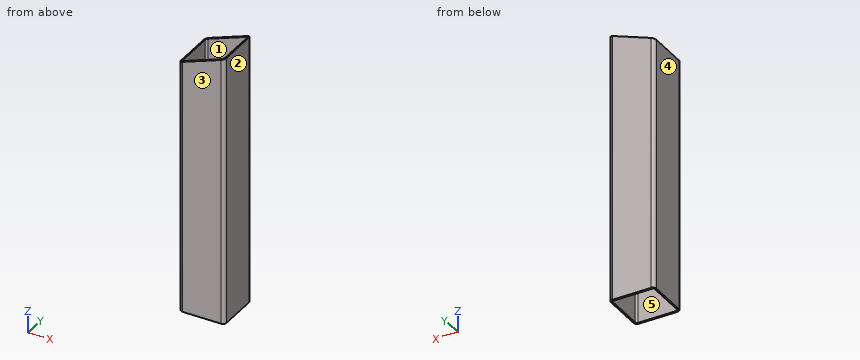
Autodesk Inventor part; units mm, degrees
ref_plane "Start plane" through (0, 0, 0) normal (0, 0, 1) x (1, 0, 0)
ref_plane "End plane" through (0, 0, 1000) normal (0, 0, 1) x (1, 0, 0)
ref_plane "YZ Plane" through (0, 0, 0) normal (1, 0, 0) x (0, 1, 0)
ref_plane "Start plane" through (0, 0, 0) normal (0, 0, 1) x (1, 0, 0)
ref_plane "End plane" through (0, 0, 1000) normal (0, 0, 1) x (1, 0, 0)
sketch "Sketch" plane through (0, 0, 0) normal (0, 0, 1) x (1, 0, 0)
  line L0 (-40, -34) -> (-40, 34)
  line L1 (-34, 40) -> (34, 40)
  line L2 (40, 34) -> (40, -34)
  line L3 (34, -40) -> (-34, -40)
  arc A0 (-40, -34) -> (-34, -40) centre (-34, -34) ccw
  arc A1 (40, 34) -> (34, 40) centre (34, 34) ccw
  arc A2 (-34, 40) -> (-40, 34) centre (-34, 34) ccw
  arc A3 (34, -40) -> (40, -34) centre (34, -34) ccw
  arc A4 (-34, 37) -> (-37, 34) centre (-34, 34) ccw
  line L4 (-34, 37) -> (34, 37)
  arc A5 (37, 34) -> (34, 37) centre (34, 34) ccw
  line L5 (37, 34) -> (37, -34)
  arc A6 (34, -37) -> (37, -34) centre (34, -34) ccw
  line L6 (34, -37) -> (-34, -37)
  arc A7 (-37, -34) -> (-34, -37) centre (-34, -34) ccw
  line L7 (-37, -34) -> (-37, 34)
  line L8 (0, 57.7397) -> (0, -57.7397) construction
  line L9 (-1453.6197, 0) -> (290.3864, 0) construction
  dimension "d7" = 6
  dimension "d9" = 80
  dimension "d11" = 80
  dimension "d12" = 3
  dimension "d15" = 40
  dimension "d16" = 40
extrude "Body" add sketch "Sketch" along normal up to surface (1000 mm away) from surface at 0
sketch "Sketch3" plane through (0, 0, 0) normal (0, 0, 1) x (1, 0, 0)
  line L0 (0, 0) -> (10, 0)
ref_plane "Work Plane3" through (0, 0, 0) normal (0, -1, 0) x (1, 0, 0)
sketch "Sketch5" plane through (0, 0, 0) normal (0, 1, 0) x (-1, 0, 0)
  line L0 (-40, 0) -> (-40, 1000)
  line L1 (40, 0) -> (40, 1000)
  line L2 (40, 0) -> (40, 1000)
  line L3 (40, 458.04) -> (415, 458.04) construction
  line L4 (-5.663, 479.3796) -> (835.663, 479.3796) construction
  arc A0 (-5.663, 479.3796) -> (415, 380) centre (415, 1320) ccw construction
  line L5 (-55, 559.2385) -> (885, 559.2385) construction
  arc A1 (-55, 559.2385) -> (-5.663, 479.3796) centre (34.3, 559.2385) ccw construction
  arc A2 (835.663, 479.3796) -> (885, 559.2385) centre (795.7, 559.2385) ccw
  line L6 (-55, 559.2385) -> (-55, 599.2385)
  line L7 (885, 559.2385) -> (885, 599.2385)
  line L8 (-55, 599.2385) -> (415, 599.2385) construction
  line L9 (415, 599.2385) -> (415, 0)
  arc A3 (415, 380) -> (835.663, 479.3796) centre (415, 1320) ccw
  line L10 (415, 599.2385) -> (885, 599.2385)
  point P0 (0, 0)
  dimension "d22" = 375
  dimension "d24" = 940
  dimension "d25" = 89.3
  dimension "d26" = 40
  dimension "d27" = 940
  dimension "d28" = 380
  dimension "d30" = 458.04
sketch "Sketch6" plane through (0, 0, 0) normal (0, 1, 0) x (-1, 0, 0)
  line L0 (40, 0) -> (40, 1000)
  line L1 (40, 0) -> (40, 1000)
  line L2 (-40, 0) -> (-40, 1000)
  line L3 (-40, 0) -> (-40, 1000)
  line L4 (34, 1000) -> (40, 1000)
  line L5 (40, 1000) -> (-40, 1000)
  arc A0 (-5.663, 479.3796) -> (415, 380) centre (415, 1320) ccw construction
  line L6 (40, 447.8824) -> (-40, 477)
  point P0 (0, 0)
  dimension "d34" = 110
  dimension "d36" = 477
extrude "Extrusion2" cut sketch "Sketch6" along normal through all both and the other way through all
sketch "Sketch4" plane through (0, 0, 0) normal (0, -1, 0) x (1, 0, 0)
  line L0 (-1453.3712, 0) -> (288.8952, 0)
  line L1 (-1453.3712, 1000) -> (288.8952, 1000)
  dimension "d18" = 1000
equation "\"d7\" = G_IR"
equation "\"d9\" = G_W"
equation "\"d11\" = G_H"
equation "\"d12\" = G_T"
equation "\"d15\" = 0.5 * d9"
equation "\"d16\" = 0.5 * d11"
equation "\"d3\" = G_L"
equation "\"d22\" = 0.5 * Diam_of_legs_center"
equation "\"d24\" = d27"
equation "\"d25\" = 0.095 * d27"
equation "\"d27\" = MAIN_filter_diam"
equation "\"G_W\" = 80"
equation "\"G_H\" = 80"
equation "\"G_T\" = 3"
equation "\"G_IR\" = 6"
equation "\"G_L\" = d18"
equation "\"G_OFFSET_START\" = 0"
equation "\"G_OFFSET_END\" = 0"
equation "\"MAIN_filter_diam\" = 940"
properties part number "SLM 1692 Leg tube" material "Steel, Mild"
Could you check a few things on this model? Use its own coordinates, in mm. Face numbers are marked on the shaded views. A direction names the side the tool comes from. Coordinates: 2 decimals unless noted, no trailing zeros. Order: outer loops, then holes, each group sorted by start corner. A loop starts at its lowest first (then second) coordinate and runs counter-clockwise, first axis right, second up. Notation, with made-up numbers: M -35,85 L 6,85 A9 ccw 6,102 Z; hole C -24,13 d6. An arc over 180 degrees is marked long. Use a Markdown table: item, result. Add a question column.
Q1. I want a section at B-B on z = 266.5. List the corners of the cut face in (x, y) for me.
Q2. Which directions (+Z, -Z, +X, -X, +Y, -Y) give clear straight access to the entire face, cutting with the end or side of a thin tool? Please do the marked faces 1 and 2.
Q3. We'd pull the mould along X, two halves only. Please class the marked faces 3, 4 and 5: pulls with the +X half, pulls with the -X half, needs draft (parallel to the pull), parting line crosses it, or undercut.
Q4. I want a section at C-C on x = 20.5. List the corners of the cut face in (y, z) for me, then the cut area to 3 significant figures.
Q5. I want a section at A-A on y = 5.5. List the corners of the cut face in (x, z) for me, then the cut area to 3 significant figures.
Q6. If I drill on L1, parallel to Y at x = -10.5, z = 312.5; L2, parallel to Y at x = 36, z = 409.5, over which ranges is the centre line in solid material (lowest first)?
Checked values:
| question | item | result |
|---|---|---|
| 1 | outline | M -40,-34 A6 ccw -34,-40 L 34,-40 A6 ccw 40,-34 L 40,34 A6 ccw 34,40 L -34,40 A6 ccw -40,34 Z; hole M -37,-34 A3 ccw -34,-37 L 34,-37 A3 ccw 37,-34 L 37,34 A3 ccw 34,37 L -34,37 A3 ccw -37,34 Z |
| 2 | face 1 | +Z, -Z |
| 2 | face 2 | +Z, -Z, +X, +Y, -Y |
| 3 | face 3 | needs draft |
| 3 | face 4 | pulls with the -X half |
| 3 | face 5 | undercut |
| 4 | outline | M -40,0 L -37,0 L -37,469.9 L -40,469.9 Z; M 37,0 L 40,0 L 40,469.9 L 37,469.9 Z |
| 4 | area | 2,820 mm² |
| 5 | outline | M -40,0 L -37,0 L -37,448.97 L -40,447.88 Z; M 37,0 L 40,0 L 40,477 L 37,475.91 Z |
| 5 | area | 2,770 mm² |
| 6 | L1 | -40 to -37, 37 to 40 |
| 6 | L2 | -39.66 to -36.24, 36.24 to 39.66 |
